```python
from build123d import *

# Parameters (mm, degrees)
F1_DEPTH = 40
F3_DEPTH = 400
F4_SIZE  = 19.99999


# Not quite as in the source:
# - a fillet or chamfer is up to 0.001 mm smaller than in the source, because OpenCascade refuses the exact size


with BuildPart() as f1:
    # F0 (on Top) → F1 (new body)
    with BuildSketch(Plane.XY):
        with BuildLine():
            Line((182.8182994574, 235.7496355578), (-177.1817005426, 235.7496355578))
            ThreePointArc((-177.1817005426, 235.7496355578), (-191.3238361663, 229.8917711815), (-197.1817005426, 215.7496355578))
            Line((-197.1817005426, 215.7496355578), (-197.1817005426, -184.2503644422))
            ThreePointArc((-197.1817005426, -184.2503644422), (-191.3238361663, -198.3925000659), (-177.1817005426, -204.2503644422))
            Line((-177.1817005426, -204.2503644422), (182.8182994574, -204.2503644422))
            ThreePointArc((182.8182994574, -204.2503644422), (196.9604350812, -198.3925000659), (202.8182994574, -184.2503644422))
            Line((202.8182994574, -184.2503644422), (202.8182994574, 215.7496355578))
            ThreePointArc((202.8182994574, 215.7496355578), (196.9604350812, 229.8917711815), (182.8182994574, 235.7496355578))
        make_face()
    extrude(amount=F1_DEPTH)

    # F2 (on face) → F3 (join)
    with BuildSketch(Plane(origin=(0, 0, 0), x_dir=(1, 0, 0), z_dir=(0, 0, -1))):
        with BuildLine():
            Line((-155.6743295648, -195.7496355578), (-132.1817005426, -195.7496355578))
            ThreePointArc((-132.1817005426, -195.7496355578), (-121.5750988248, -191.3562372756), (-117.1817005426, -180.7496355578))
            Line((-117.1817005426, -180.7496355578), (-117.1817005426, -170.7496355578))
            ThreePointArc((-117.1817005426, -170.7496355578), (-121.5750988248, -160.14303384), (-132.1817005426, -155.7496355578))
            Line((-132.1817005426, -155.7496355578), (-142.1817005426, -155.7496355578))
            ThreePointArc((-142.1817005426, -155.7496355578), (-152.7883022604, -160.14303384), (-157.1817005426, -170.7496355578))
            Line((-157.1817005426, -170.7496355578), (-157.1817005426, -194.2422645801))
            ThreePointArc((-157.1817005426, -194.2422645801), (-156.740201805, -195.3081368202), (-155.6743295648, -195.7496355578))
        make_face()
        with BuildLine():
            Line((124.3256704352, -195.7496355578), (147.8182994574, -195.7496355578))
            ThreePointArc((147.8182994574, -195.7496355578), (158.4249011752, -191.3562372756), (162.8182994574, -180.7496355578))
            Line((162.8182994574, -180.7496355578), (162.8182994574, -170.7496355578))
            ThreePointArc((162.8182994574, -170.7496355578), (158.4249011752, -160.14303384), (147.8182994574, -155.7496355578))
            Line((147.8182994574, -155.7496355578), (137.8182994574, -155.7496355578))
            ThreePointArc((137.8182994574, -155.7496355578), (127.2116977396, -160.14303384), (122.8182994574, -170.7496355578))
            Line((122.8182994574, -170.7496355578), (122.8182994574, -194.2422645801))
            ThreePointArc((122.8182994574, -194.2422645801), (123.259798195, -195.3081368202), (124.3256704352, -195.7496355578))
        make_face()
        with BuildLine():
            Line((124.3256704352, 124.2503644422), (147.8182994574, 124.2503644422))
            ThreePointArc((147.8182994574, 124.2503644422), (158.4249011752, 128.6437627244), (162.8182994574, 139.2503644422))
            Line((162.8182994574, 139.2503644422), (162.8182994574, 149.2503644422))
            ThreePointArc((162.8182994574, 149.2503644422), (158.4249011752, 159.85696616), (147.8182994574, 164.2503644422))
            Line((147.8182994574, 164.2503644422), (137.8182994574, 164.2503644422))
            ThreePointArc((137.8182994574, 164.2503644422), (127.2116977396, 159.85696616), (122.8182994574, 149.2503644422))
            Line((122.8182994574, 149.2503644422), (122.8182994574, 125.7577354199))
            ThreePointArc((122.8182994574, 125.7577354199), (123.259798195, 124.6918631798), (124.3256704352, 124.2503644422))
        make_face()
        with BuildLine():
            Line((-155.6743295648, 124.2503644422), (-132.1817005426, 124.2503644422))
            ThreePointArc((-132.1817005426, 124.2503644422), (-121.5750988248, 128.6437627244), (-117.1817005426, 139.2503644422))
            Line((-117.1817005426, 139.2503644422), (-117.1817005426, 149.2503644422))
            ThreePointArc((-117.1817005426, 149.2503644422), (-121.5750988248, 159.85696616), (-132.1817005426, 164.2503644422))
            Line((-132.1817005426, 164.2503644422), (-142.1817005426, 164.2503644422))
            ThreePointArc((-142.1817005426, 164.2503644422), (-152.7883022604, 159.85696616), (-157.1817005426, 149.2503644422))
            Line((-157.1817005426, 149.2503644422), (-157.1817005426, 125.7577354199))
            ThreePointArc((-157.1817005426, 125.7577354199), (-156.740201805, 124.6918631798), (-155.6743295648, 124.2503644422))
        make_face()
    extrude(amount=F3_DEPTH)

    # F4 (size 20 in the source; OpenCascade refuses exactly that, so slightly less here)
    f4_edges = [f1.edges().sort_by_distance(p)[0] for p in [
        (2.818299, 235.749636, 40),
        (-191.323836, 229.891771, 40),
        (-197.181701, 15.749636, 40),
        (-191.323836, -198.3925, 40),
        (2.818299, -204.250364, 40),
        (196.960435, -198.3925, 40),
        (202.818299, 15.749636, 40),
        (196.960435, 229.891771, 40),
    ]]
    chamfer(f4_edges, length=F4_SIZE)


solid = f1.part
```
Here's how the part is built. I have some questions about the finished solid (model axes, mm). A direction names the side the tool comes from. Coordinates: 2 decimals unless noted, no trailing zeros. Write each loop counter-clockwise with the first axis right and the second up, starting at its lowest first coordinate (ties: lowest second). Pieces come first, ordered by that corner, then holes. Notation, with made-up numbers: (76.25, -17) -> (108.25, -17) arc R26 cw to (108.25, 12) -> close; hole circle Ø5 at (-38, -3). An arc over 180 degrees is marked (long way). Use a Markdown table: item, result. Add a question column.
(1) I'm going to push flat-ended pins straight in: P1, Ø11, axis at y = 177, z = -168.5, coming from the +X side; P2, Ø3, axis at x = -138.5, z = -126, coming from the -Y side; P3, Ø19, axis at x = -142.5, z = -195.5, coming from the +Y side. Where does each tip first touch, or does it pass through?
(2) For faces 1 (the cylindrical face through (127.329, 160.027, -197.2)), 2 (the flat face through (136, 195.75, -197)), 3 (the cylindrical face through (-121.46, -159.74, -197.2)), which set-ups out of +Z, -Z, +X, -X, +Y, -Y let a thin tool reach every point of the face, with its end or its side?
(3) If we section it at C-C, the plane y = -8.5: Write out the boundary of the cut face in (x, z).
(4) Please list where these lines run through material, in increasing order: line 1 (X direction, y = -146.5, z = -189.5); line 2 (Z direction, x = 129.5, y = 105); line 3 (Y direction, x = -121, z = -80).
(5) We'd pull the mould along Y, two halves only. Please class faces 4 (the flat face through (5, 235.75, 10)), 5 (the cylindrical face through (-191.478, -198.236, 9.86)), 6 (the flat face through (-144, -124.25, -197)): +Y half, -Y half, draft (parallel to the pull), parting line (faces both ways), or undercut.
(6) If we section it at B-B, the plane x = 72: Write out the boundary of the cut face in (y, z), and give its area (3 significant figures).
(7) If we section it at A-A, the plane z = -165: State how many separate pieces and enclosed holes the cut face has, and give its area (3 significant figures).
Outcome:
| question | item | result |
|---|---|---|
| 1 | P1 | stops at x = 162.82 |
| 1 | P2 | stops at y = -164.25 |
| 1 | P3 | stops at y = 195.75 |
| 2 | face 1 | -Z |
| 2 | face 2 | -Z, +X, -X, +Y |
| 2 | face 3 | -Z, -Y |
| 3 | outline | (-197.18, 0) -> (202.82, 0) -> (202.82, 20) -> (182.82, 40) -> (-177.18, 40) -> (-197.18, 20) -> close |
| 4 | line 1 | x = -157.18 to -117.18, 122.82 to 162.82 |
| 4 | line 2 | z = 0 to 40 |
| 4 | line 3 | y = -159.25 to -129.25, 160.75 to 190.75 |
| 5 | face 4 | +Y half |
| 5 | face 5 | -Y half |
| 5 | face 6 | undercut |
| 6 | outline | (-204.25, 0) -> (235.75, 0) -> (235.75, 20) -> (215.75, 40) -> (-184.25, 40) -> (-204.25, 20) -> close |
| 6 | area | 17,200 mm^2 |
| 7 | separate pieces | 4 |
| 7 | enclosed holes | 0 |
| 7 | area | 5,820 mm^2 |
